```python
from build123d import *

# Parameters (mm, degrees)
SKETCH4_R           = 10.7188
BOSS_EXTRUDE1_DEPTH = 6.63575
SKETCH5_W           = 6.63575
SKETCH5_H           = 0.254


with BuildPart() as part:
    # Sketch3 → Revolve1 (revolve)
    with BuildSketch(Plane(origin=(0, 0, 0), x_dir=(0, 0, -1), z_dir=(1, 0, 0))):
        with BuildLine():
            Line((6.461125, 0), (13.096875, 0))
            Line((13.096875, 0), (13.096875, -10.7188))
            Line((13.096875, -10.7188), (-13.096875, -10.7188))
            Line((-13.096875, -10.7188), (-13.096875, -7.9502))
            Line((-13.096875, -7.9502), (4.873625, -7.9502))
            ThreePointArc((4.873625, -7.9502), (6.060370876, -4.053573618), (6.461125, 0))
        make_face()
    revolve(axis=Axis((0, 0, 13.096875), (0, 0, -1)))

    # Sketch4 → Boss-Extrude1 (add)
    with BuildSketch(Plane(origin=(0, 0, -13.096875), x_dir=(-1, 0, 0), z_dir=(0, 0, -1))):
        Polygon((4.99748663, 12.065), (-4.99748663, 12.065), (-12.065, 4.99748663), (-12.065, -4.99748663), (-4.99748663, -12.065), (4.99748663, -12.065), (12.065, -4.99748663), (12.065, 4.99748663), align=None)
        Circle(SKETCH4_R, mode=Mode.SUBTRACT)
    extrude(amount=-BOSS_EXTRUDE1_DEPTH)

    # Sketch5 → Cut-Revolve1 (revolve, cut)
    with BuildSketch(Plane(origin=(0, 0, 0), x_dir=(0, 0, -1), z_dir=(0.923879533, -0.382683432, 0))):
        with Locations((9.779, 12.932061897)):
            Rectangle(SKETCH5_W, SKETCH5_H)
    revolve(axis=Axis((0, 0, 13.096875), (0, 0, 1)), mode=Mode.SUBTRACT)


solid = part.part
```
The listing builds one solid part. Answer for the finished solid, in the listing's coordinates (mm). A direction names the side the tool comes from. Give positions to 0.01 mm unless a question says otherwise; leave off trailing zeros. Write each loop counter-clockwise with the first axis right and the second up, starting at its lowest first coordinate (ties: lowest second). Pieces come first, ordered by that corner, then holes. Notation, with made-up numbers: M 62,27.5 L 91,27.5 A19 cw 91,50.5 Z; hole C 78,-34.75 d9. An arc over 180 degrees is marked long. Write each question's results on one line, items separated by ' | '.
Q1. Consider L1, parallel to Y at x = 0, z = 7.5; L2, parallel to Y at x = -6, z = 6.75. Determine where each line is inside the solid, lowest interval first. Write a range as from..to.
Output values:
L1: -10.72..-7.95, 7.95..10.72 | L2: -8.88..-5.22, 5.22..8.88
Q2. Section A-A, the plane x = 0 is taken. Write down the section's boundary in (y, z) (3 decimals), then the cut area to 3 significant figures.
Output values:
outline: M -12.065,-13.097 L 12.065,-13.097 L 12.065,-6.461 L 10.719,-6.461 L 10.719,13.097 L 7.95,13.097 L 7.95,-4.874 A20.701 cw -7.95,-4.874 L -7.95,13.097 L -10.719,13.097 L -10.719,-6.461 L -12.065,-6.461 Z | area: 277 mm2
Q3. For a pull along X with two mould halves and no side action, classify faces 1 (the cylindrical face through (7.76, 1.72, 3.99)), 2 (the cylindrical face through (11.834, 4.892, -9.825)), 3 (the cylindrical face through (-4.892, 11.834, -9.825)) as released by +X, released by -X, zero draft, split by the parting line, or undercut.
Output values:
face 1: undercut | face 2: released by +X | face 3: released by -X
Q4. A tool of negligible diameter and unlimited length cuts with its end or side. For faces 4 (the cylindrical face through (4.11, -9.9, 3.45)), 5 (the cylindrical face through (4.892, -11.834, -9.825)), from which of +Z, -Z, +X, -X, +Y, -Y can it reach the whole face along a straight path? Write none if from no direction.
Output values:
face 4: +Z | face 5: +Z, -Z, +X, -Y
Q5. Section C-C, the plane z = 9.5 is taken. Write down the section's boundary in (x, y), then the cut area to 3 significant figures.
Output values:
outline: C 0,0 d21.44; hole C 0,0 d15.9 | area: 162 mm2
Q6. Flat-ended cylindrical pins translate along their axes: P1, Ø4, axis at x = -9.5, z = -3.5, coming from the +Y side; P2, Ø1.5, axis at x = -8, y = 9.5, coming from the +Z side; P3, Ø12, axis at y = -0.5, z = 6, coming from the -X side. Find the tip coordinate at first contact, or state that the pin passes through.
Output values:
P1: y = 7.66 | P2: z = -6.46 | P3: x = -10.72
